```python
from build123d import *

# Parameters (mm, degrees)
CUT_EXTRUDE1_START = 2.2987
CUT_EXTRUDE1_DEPTH = 10.922
CIRPATTERN1_COUNT  = 10
SKETCH4_R          = 1.190625
CUT_EXTRUDE2_DEPTH = 19.796832346
CUT_EXTRUDE3_DEPTH = 0.89296875
CIRPATTERN2_COUNT  = 2
CIRPATTERN2_ANGLE  = 90


with BuildPart() as part:
    # Sketch2 → Revolve1 (revolve)
    with BuildSketch(Plane(origin=(0, 0, 0), x_dir=(0, 0, -1), z_dir=(1, 0, 0)), mode=Mode.PRIVATE) as revolve1_sk:
        with BuildLine():
            Line((-10.3124, 2.38125), (10.3124, 2.38125))
            Line((10.3124, 2.38125), (10.3124, 11.1125))
            Line((10.3124, 11.1125), (9.46785, 11.1125))
            ThreePointArc((9.46785, 11.1125), (8.84593021, 10.355304295), (8.6233, 9.401068816))
            Line((8.6233, 9.401068816), (8.6233, 7.689637631))
            Line((8.6233, 7.689637631), (-2.2987, 7.689637631))
            Line((-2.2987, 7.689637631), (-2.2987, 9.401068816))
            ThreePointArc((-2.2987, 9.401068816), (-2.52133021, 10.355304295), (-3.14325, 11.1125))
            Line((-3.14325, 11.1125), (-3.9878, 11.1125))
            Line((-3.9878, 11.1125), (-3.9878, 5.5499))
            Line((-3.9878, 5.5499), (-10.3124, 5.5499))
            Line((-10.3124, 5.5499), (-10.3124, 2.38125))
        make_face()
    revolve(revolve1_sk.sketch.rotate(Axis((0, 0, 10.3124), (0, 0, -1)), 90), axis=Axis((0, 0, 10.3124), (0, 0, -1)))

    # Sketch3 → Cut-Extrude1 (cut)
    with BuildSketch(Plane.XY.offset(CUT_EXTRUDE1_START)):
        with BuildLine():
            Line((-0.690489274, 6.3119), (0.690489274, 6.3119))
            Line((0.690489274, 6.3119), (1.2827, 7.5819))
            ThreePointArc((1.2827, 7.5819), (0, 7.689637631), (-1.2827, 7.5819))
            Line((-1.2827, 7.5819), (-0.690489274, 6.3119))
        make_face()
    cut_extrude1 = extrude(amount=-CUT_EXTRUDE1_DEPTH, mode=Mode.SUBTRACT)

    # CirPattern1: Cut-Extrude1 ×10 about axis
    cirpattern1_axis = Axis((0, 0, 0), (0, 0, 1))
    for i in range(1, CIRPATTERN1_COUNT):
        add(cut_extrude1.rotate(cirpattern1_axis, i * 360 / CIRPATTERN1_COUNT), mode=Mode.SUBTRACT)

    # Sketch4 → Cut-Extrude2 (cut, through all)
    with BuildSketch(Plane(origin=(0, 0, 0), x_dir=(1, 0, 0), z_dir=(0, 1, 0))):
        with Locations(Location((0, -7.1501, 0), (0, 0, 90))):
            Circle(SKETCH4_R)
    cut_extrude2 = extrude(amount=CUT_EXTRUDE2_DEPTH, mode=Mode.SUBTRACT)

    # Sketch5 → Revolve2 (revolve)
    with BuildSketch(Plane.XY.offset(7.1501), mode=Mode.PRIVATE) as revolve2_sk:
        Polygon((0, 5.420682809), (0, 2.38125), (-0.555625, 2.38125), (-1.190625, 3.01625), (-1.190625, 4.785682809), (-0.555625, 5.420682809), align=None)
    revolve2 = revolve(revolve2_sk.sketch.rotate(Axis((0, 0, 7.1501), (0, 1, 0)), 270), axis=Axis((0, 0, 7.1501), (0, 1, 0)))

    # Sketch6 → Cut-Extrude3 (cut)
    with BuildSketch(Plane(origin=(0, 5.420682809, 0), x_dir=(-1, 0, 0), z_dir=(0, -1, 0))):
        Polygon((0, -6.462692336), (-0.5953125, -6.806396168), (-0.5953125, -7.493803832), (0, -7.837507664), (0.5953125, -7.493803832), (0.5953125, -6.806396168), align=None)
    cut_extrude3 = extrude(amount=CUT_EXTRUDE3_DEPTH, mode=Mode.SUBTRACT)

    # CirPattern2: Cut-Extrude2, Revolve2, Cut-Extrude3 ×2 about axis
    cirpattern2_axis = Axis((0, 0, 0), (0, 0, -1))
    add([cut_extrude2.rotate(cirpattern2_axis, i * CIRPATTERN2_ANGLE / (CIRPATTERN2_COUNT - 1)) for i in range(1, CIRPATTERN2_COUNT)], mode=Mode.SUBTRACT)
    add([revolve2.rotate(cirpattern2_axis, i * CIRPATTERN2_ANGLE / (CIRPATTERN2_COUNT - 1)) for i in range(1, CIRPATTERN2_COUNT)])
    add([cut_extrude3.rotate(cirpattern2_axis, i * CIRPATTERN2_ANGLE / (CIRPATTERN2_COUNT - 1)) for i in range(1, CIRPATTERN2_COUNT)], mode=Mode.SUBTRACT)


solid = part.part
```
The listing builds one solid part. Answer for the finished solid, in the listing's coordinates (mm). A direction names the side the tool comes from. Give positions to 0.01 mm unless a question says otherwise; leave off trailing zeros. Order: outer loops, then holes, each group sorted by start corner. A loop starts at its lowest first (then second) coordinate and runs counter-clockwise, first axis right, second up. Notation, with made-up numbers: M 38,-2 L 47,-2 A30 cw 47,34 Z; hole C 72.5,75.5 d9. An arc over 180 degrees is marked long. Put each result on its own line as item: value. Start each with the question number.
Item 1: Flat-ended cylindrical pins translate along their axes: P1, Ø0.8, axis at y = 5, z = 7, coming from the -X side; P2, Ø1.5, axis at y = 3, z = -3.5, coming from the +X side; P3, Ø10, axis at x = 6, z = -3.5, coming from the -Y side. Find the tip coordinate at first contact, or state that the pin passes through.
Item 2: The part is cut by section A-A, the plane z = 5. Determine the outline of the cut face in (x, y).
Item 3: Which of the six approach directions +Z, -Z, +X, -X, +Y, -Y give full straight-line access (tool end or side, diameter ignored) to faces 1 (the face through (-3.72, 5.1, -3.09)), 2 (the face through (6.9, 1.21, -3.09)), 3 (the face through (-6.31, -3.09, -3.09)), 4 (the face through (-4.873, -5.035, -3.086))?
Item 4: For a pull along Y with two mould halves and no side action, classify faces 5 (the face through (-8.2, -7.5, -9.9)), 6 (the face through (2.36, 7.32, -3.09)), 7 (the face through (-6.006, 1.941, -3.086)) as +Y half, -Y half, draft (parallel to the pull), parting line (faces both ways), or undercut.
Item 5: Find the intervals of material crossed by line 1 along Z through (x, y) = (7, 1.5); line 2 along Y through (x, z) = (0, -5.5); line 3 along X through (y, z) = (-3, 2.25), in increasing order.
Answer key:
1. P1: stops at x = -3.11
1. P2: stops at x = 6.81
1. P3: stops at y = -7.58
2. outline: C 0,0 d11.1; hole C 0,0 d4.76
3. face 1: none
3. face 2: +X
3. face 3: -X
3. face 4: -Y
4. face 5: parting line
4. face 6: +Y half
4. face 7: undercut
5. line 1: z = -10.31 to -8.62, 2.3 to 3.99
5. line 2: y = -6.31 to -2.38, 2.38 to 6.31
5. line 3: x = -6.21 to 6.21
